The model under review builds one solid part; all positions refer to its coordinate system, in mm. Face numbers are marked on the shaded views. A direction names the side the tool comes from. Give positions to 0.01 mm unless a question says otherwise; leave off trailing zeros. Order: outer loops, then holes, each group sorted by start corner. A loop starts at its lowest first (then second) coordinate and runs counter-clockwise, first axis right, second up. Notation, with made-up numbers: (-9, 27) - (29, 27) arc R25 ccw to (29, 42) - close; hole circle Ø6 at (-15, 69.5). An arc over 180 degrees is marked (long way). Use a Markdown table: item, result. Add a question column.
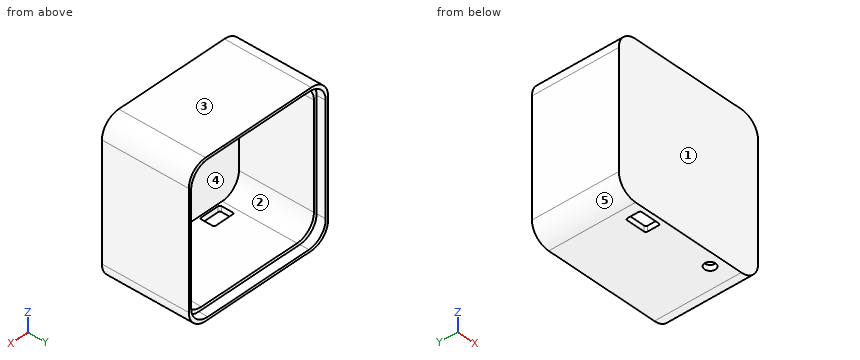
```python
from build123d import *

# Parameters (mm, degrees)
BOSS_EXTRUDE1_DEPTH = 46
CUT_EXTRUDE1_DEPTH  = 5
BOSS_EXTRUDE2_START = 1.5
BOSS_EXTRUDE2_DEPTH = 1.5
SKETCH4_R           = 3
CUT_EXTRUDE2_DEPTH  = 8


with BuildPart() as part:
    # Sketch1 → Boss-Extrude1 (new body)
    with BuildSketch(Plane(origin=(0, 0, 0), x_dir=(1, 0, 0), z_dir=(0, 1, 0))):
        with BuildLine():
            Line((-31.5, 41.5), (31.5, 41.5))
            ThreePointArc((31.5, 41.5), (38.571067812, 38.571067812), (41.5, 31.5))
            Line((41.5, 31.5), (41.5, -31.5))
            ThreePointArc((41.5, -31.5), (38.571067812, -38.571067812), (31.5, -41.5))
            Line((31.5, -41.5), (-31.5, -41.5))
            ThreePointArc((-31.5, -41.5), (-38.571067812, -38.571067812), (-41.5, -31.5))
            Line((-41.5, -31.5), (-41.5, 31.5))
            ThreePointArc((-41.5, 31.5), (-38.571067812, 38.571067812), (-31.5, 41.5))
        make_face()
        with BuildLine():
            Line((-28.5, 38.5), (28.5, 38.5))
            ThreePointArc((28.5, 38.5), (35.571067812, 35.571067812), (38.5, 28.5))
            Line((38.5, 28.5), (38.5, -28.5))
            ThreePointArc((38.5, -28.5), (35.571067812, -35.571067812), (28.5, -38.5))
            Line((28.5, -38.5), (-28.5, -38.5))
            ThreePointArc((-28.5, -38.5), (-35.571067812, -35.571067812), (-38.5, -28.5))
            Line((-38.5, -28.5), (-38.5, 28.5))
            ThreePointArc((-38.5, 28.5), (-35.571067812, 35.571067812), (-28.5, 38.5))
        make_face(mode=Mode.SUBTRACT)
    extrude(amount=BOSS_EXTRUDE1_DEPTH)

    # Sketch2 → Cut-Extrude1 (cut)
    with BuildSketch(Plane(origin=(0, 46, 0), x_dir=(1, 0, 0), z_dir=(0, 1, 0))):
        with BuildLine():
            Line((-30.1, 40.1), (30.1, 40.1))
            ThreePointArc((30.1, 40.1), (37.171067812, 37.171067812), (40.1, 30.1))
            Line((40.1, 30.1), (40.1, -30.1))
            ThreePointArc((40.1, -30.1), (37.171067812, -37.171067812), (30.1, -40.1))
            Line((30.1, -40.1), (-30.1, -40.1))
            ThreePointArc((-30.1, -40.1), (-37.171067812, -37.171067812), (-40.1, -30.1))
            Line((-40.1, -30.1), (-40.1, 30.1))
            ThreePointArc((-40.1, 30.1), (-37.171067812, 37.171067812), (-30.1, 40.1))
        make_face()
    extrude(amount=-CUT_EXTRUDE1_DEPTH, mode=Mode.SUBTRACT)

    # Sketch3 → Boss-Extrude2 (add)
    with BuildSketch(Plane.XZ.offset(BOSS_EXTRUDE2_START)):
        with BuildLine():
            Line((-31.5, 41.5), (31.5, 41.5))
            ThreePointArc((31.5, 41.5), (38.571067812, 38.571067812), (41.5, 31.5))
            Line((41.5, 31.5), (41.5, -31.5))
            ThreePointArc((41.5, -31.5), (38.571067812, -38.571067812), (31.5, -41.5))
            Line((31.5, -41.5), (-31.5, -41.5))
            ThreePointArc((-31.5, -41.5), (-38.571067812, -38.571067812), (-41.5, -31.5))
            Line((-41.5, -31.5), (-41.5, 31.5))
            ThreePointArc((-41.5, 31.5), (-38.571067812, 38.571067812), (-31.5, 41.5))
        make_face()
    extrude(amount=-BOSS_EXTRUDE2_DEPTH)

    # Sketch4 → Cut-Extrude2 (cut)
    with BuildSketch(Plane(origin=(0, 0, -41.5), x_dir=(-1, 0, 0), z_dir=(0, 0, -1))):
        with Locations((-20, 5)):
            Circle(SKETCH4_R)
        with BuildLine():
            Line((15, 1), (25, 1))
            ThreePointArc((25, 1), (25.707106781, 1.292893219), (26, 2))
            Line((26, 2), (26, 8))
            ThreePointArc((26, 8), (25.707106781, 8.707106781), (25, 9))
            Line((25, 9), (15, 9))
            ThreePointArc((15, 9), (14.292893219, 8.707106781), (14, 8))
            Line((14, 8), (14, 2))
            ThreePointArc((14, 2), (14.292893219, 1.292893219), (15, 1))
        make_face()
    extrude(amount=-CUT_EXTRUDE2_DEPTH, mode=Mode.SUBTRACT)


solid = part.part
```
Q1. We need section B-B (y = 5). Write out the cut boundary in (x, z), plus the area to 3 significant figures.
Q2. Wall thickness on probe 1 along X at (y, z) = (35, 7); probe 2 along Y at (x, z) = (20, -40): over which ranges is each line inside the solid? List them lowest first.
Q3. Clearance check with flat-ended pins moving along their axes: P1, Ø1.5, axis at y = 6, z = -40.5, coming from the +X side; P2, Ø2.5, axis at y = 4, z = -39.5, coming from the -X side; P3, Ø4, axis at x = 21, z = 3.5, coming from the +Y side. State where each tip first meets the part, or that it passes through.
Q4. Machinability: for the marked faces 4 and 5, which of the approach directions +Z, -Z, +X, -X, +Y, -Y give a long, thin tool a straight path to every point of the face, cutting with its end or side? Answer none if there is none.
Q5. We need section D-D (y = 35). Write out the cut boundary in (x, z).
Q6. We need section A-A (x = 20). Write out the cut boundary in (y, z).
Q7. Draft analysis for pull direction Z (two halves, no side actions). For the marked faces 1, 2 and 3, state which applies: pulls with the +Z half, pulls with the -Z half, needs draft (parallel to the pull), parting line crosses it, or undercut.
Q8. We need section C-C (x = 10). Write out the cut boundary in (y, z), plus the area to 4 significant figures.
Here are the results:
| question | item | result |
|---|---|---|
| 1 | outline | (-41.5, -31.5) arc R10 ccw to (-31.5, -41.5) - (-26, -41.5) - (-26, -38.5) - (-28.5, -38.5) arc R10 cw to (-38.5, -28.5) - (-38.5, 28.5) arc R10 cw to (-28.5, 38.5) - (28.5, 38.5) arc R10 cw to (38.5, 28.5) - (38.5, -28.5) arc R10 cw to (28.5, -38.5) - (23, -38.5) - (23, -41.5) - (31.5, -41.5) arc R10 ccw to (41.5, -31.5) - (41.5, 31.5) arc R10 ccw to (31.5, 41.5) - (-31.5, 41.5) arc R10 ccw to (-41.5, 31.5) - close; (-14, -41.5) - (17, -41.5) - (17, -38.5) - (-14, -38.5) - close |
| 1 | area | 906 mm2 |
| 2 | probe 1 | -41.5 to -38.5, 38.5 to 41.5 |
| 2 | probe 2 | -1.5 to 2, 8 to 41 |
| 3 | P1 | x = 37.15 |
| 3 | P2 | x = -38.88 |
| 3 | P3 | y = 0 |
| 4 | face 4 | +Y |
| 4 | face 5 | -Z, -X, +Y, -Y |
| 5 | outline | (-41.5, -31.5) arc R10 ccw to (-31.5, -41.5) - (31.5, -41.5) arc R10 ccw to (41.5, -31.5) - (41.5, 31.5) arc R10 ccw to (31.5, 41.5) - (-31.5, 41.5) arc R10 ccw to (-41.5, 31.5) - close; hole (-38.5, -28.5) arc R10 ccw to (-28.5, -38.5) - (28.5, -38.5) arc R10 ccw to (38.5, -28.5) - (38.5, 28.5) arc R10 ccw to (28.5, 38.5) - (-28.5, 38.5) arc R10 ccw to (-38.5, 28.5) - close |
| 6 | outline | (-1.5, -41.5) - (2, -41.5) - (2, -38.5) - (0, -38.5) - (0, 38.5) - (41, 38.5) - (41, 40.1) - (46, 40.1) - (46, 41.5) - (-1.5, 41.5) - close; (8, -41.5) - (46, -41.5) - (46, -40.1) - (41, -40.1) - (41, -38.5) - (8, -38.5) - close |
| 7 | face 1 | needs draft |
| 7 | face 2 | undercut |
| 7 | face 3 | pulls with the +Z half |
| 8 | outline | (-1.5, -41.5) - (46, -41.5) - (46, -40.1) - (41, -40.1) - (41, -38.5) - (0, -38.5) - (0, 38.5) - (41, 38.5) - (41, 40.1) - (46, 40.1) - (46, 41.5) - (-1.5, 41.5) - close |
| 8 | area | 384.5 mm2 |
